from build123d import *

# Parameters (mm, degrees)
F0_W     = 56
F0_H     = 110
F1_DEPTH = 5
F2_W     = 6
F2_H     = 32
F2_W_2   = 22.5
F2_H_2   = 11.8
F2_R     = 2.885
F2_R_2   = 2.5
F3_DEPTH = 25


with BuildPart() as f1:
    # F0 (on Front) → F1 (new body)
    with BuildSketch(Plane.XZ):
        with Locations((-15.773296, 12.593315)):
            Rectangle(F0_W, F0_H)
    extrude(amount=F1_DEPTH)

    # F2 (on face) → F3 (cut)
    with BuildSketch(Plane.XZ.offset(5)):
        with Locations((-2.773296, -26.406685)):
            Rectangle(F2_W, F2_H)
        with Locations((-28.773296, -26.406685)):
            Rectangle(F2_W, F2_H)
        with Locations((-16.29366, 45.039438)):
            Rectangle(F2_W_2, F2_H_2)
        with Locations((-32.292966, 28.889665)):
            Circle(F2_R)
        with Locations((-32.292966, 10.118715)):
            Circle(F2_R_2)
    extrude(amount=-F3_DEPTH, mode=Mode.SUBTRACT)


solid = f1.part
The listing builds one solid part. Answer for the finished solid, in the listing's coordinates (mm). A direction names the side the tool comes from. Give positions to 0.01 mm unless a question says otherwise; leave off trailing zeros. Write each loop counter-clockwise with the first axis right and the second up, starting at its lowest first coordinate (ties: lowest second). Pieces come first, ordered by that corner, then holes.
Item 1: Flat-ended cylindrical pins translate along their axes: P1, Ø4.5, axis at x = -32.29, z = 28.89, coming from the +Y side; P2, Ø1.5, axis at x = -2, y = -2, coming from the -Z side. Find the tip coordinate at first contact, or state that the pin passes through.
Item 2: Find the intervals of material crossed by line 1 along X through (y, z) = (-0.7, -34); line 2 along X through (y, z) = (-3.25, 48); line 3 along Z through (x, y) = (-25, -3.95), in increasing order.
Item 3: Section D-D, the plane y = -3.7 is taken. Write down the section's boundary in (x, z) (3 decimals), plus the area to 3 significant figures.
Item 4: Section A-A, the plane x = -16.5 is taken. Write down the section's boundary in (y, z).
Item 5: Section C-C, the plane z = 42 is taken. Write down the section's boundary in (x, y), plus the area to 4 significant figures.
Item 6: Which of the six approach directions +Z, -Z, +X, -X, +Y, -Y give full straight-line access (tool end or side, diameter ignored) to faces 1 (the flat face through (0.227, -3, -27)), 2 (the flat face through (-16, -3, 50.939)), 3 (the flat face through (-16, 0, 13))?
Item 7: Section B-B, the plane z = -22 is taken. Write down the section's boundary in (x, y), plus the area to 3 significant figures.
Item 8: Determine the mould class of faces 4 (the flat face through (12.227, -2, 12)), 5 (the flat face through (-5.773, -3, -27)), 6 (the flat face through (-16, -2, 67.593)) for opening direction X: released by +X, released by -X, zero draft, split by the parting line, or undercut.
Completed:
1. P1: passes through
1. P2: stops at z = -10.41
2. line 1: x = -43.77 to -31.77, -25.77 to -5.77, 0.23 to 12.23
2. line 2: x = -43.77 to -27.54, -5.04 to 12.23
2. line 3: z = -42.41 to 39.14, 50.94 to 67.59
3. outline: (-43.773, -42.407) - (-31.773, -42.407) - (-31.773, -10.407) - (-25.773, -10.407) - (-25.773, -42.407) - (-5.773, -42.407) - (-5.773, -10.407) - (0.227, -10.407) - (0.227, -42.407) - (12.227, -42.407) - (12.227, 67.593) - (-43.773, 67.593) - close; hole circle Ø5.77 at (-32.293, 28.89); hole circle Ø5 at (-32.293, 10.119); hole (-27.544, 39.139) - (-5.044, 39.139) - (-5.044, 50.939) - (-27.544, 50.939) - close
3. area: 5,460 mm2
4. outline: (-5, -42.41) - (0, -42.41) - (0, 39.14) - (-5, 39.14) - close; (-5, 50.94) - (0, 50.94) - (0, 67.59) - (-5, 67.59) - close
5. outline: (-43.77, -5) - (-27.54, -5) - (-27.54, 0) - (-43.77, 0) - close; (-5.04, -5) - (12.23, -5) - (12.23, 0) - (-5.04, 0) - close
5. area: 167.5 mm2
6. face 1: -Z, +Y, -Y
6. face 2: +Y, -Y
6. face 3: +Z, -Z, +X, -X, +Y
7. outline: (-43.77, -5) - (-31.77, -5) - (-31.77, 0) - (-43.77, 0) - close; (-25.77, -5) - (-5.77, -5) - (-5.77, 0) - (-25.77, 0) - close; (0.23, -5) - (12.23, -5) - (12.23, 0) - (0.23, 0) - close
7. area: 220 mm2
8. face 4: released by +X
8. face 5: undercut
8. face 6: zero draft
